Geometry: final body of the model. Coordinates: model frame, mm. Face numbers are marked on the shaded views. A direction names the side the tool comes from. Give positions to 0.01 mm unless a question says otherwise; leave off trailing zeros. Write each loop counter-clockwise with the first axis right and the second up, starting at its lowest first coordinate (ties: lowest second). Pieces come first, ordered by that corner, then holes.
Q1. Section A-A (x = 60.5). Return the cut outline in (y, z), plus the area to 3 significant figures.
Q2. Line query: line 1 (Y direction, x = 60.5, z = 2.9); line 2 (X direction, y = -88.6, z = -52.57); line 3 (Z direction, x = 18.5, y = -48). Output: solid intervals per line, ascending.
Q3. Mould query, pull axis Z, two halves, no side actions, for the marked faces 4, 5 and 6. Classes: +Z half, -Z half, draft (parallel to the pull), parting line (faces both ways), or undercut.
Q4. Pin query (flat end, axial travel): pin 1 Ø4 at (y, z) = (-19, 3.5) entering from -X; pin 2 Ø1.5 at (x, y) = (25, -57) entering from -Z; pin 3 Ø9.5 at (x, z) = (42, -31.5) entering from -Y; pin 4 Ø6.5 at (x, y) = (60.5, -22.94) entering from -Z. Return the tip coordinate at first contact, or that it passes through.
Q5. Reachability of the marked faces 1, 2 and 3 from +Z, -Z, +X, -X, +Y, -Y: full face, straight path, thin tool, end or side. Return the list, or none.
Q6. Section D-D (y = -50.5). Return the cut outline in (x, z).
Q7. Section C-C (y = -35.5). Return the cut outline in (x, z).
Q8. Section B-B (z = -21.66). Return the cut outline in (x, y).
from build123d import *

# Parameters (mm, degrees)
BOSS_EXTRUDE1_DEPTH   = 5
SKETCH2_W             = 6.35
SKETCH2_H             = 50
BOSS_EXTRUDE2_DEPTH   = 52.48
CUT_EXTRUDE1_REACH    = 106.448
SKETCH3_R             = 20.44
SKETCH3_R_2           = 2.555
SKETCH3_W             = 5
SKETCH3_H             = 50
CUT_EXTRUDE2_REACH    = 108.104
SKETCH4_R             = 3.5
CUT_EXTRUDE6_REACH    = 108.104
SKETCH14_W            = 23.196263878
SKETCH14_H            = 15.316152196
SKETCH15_W            = 12
SKETCH15_H            = 3.2
BOSS_EXTRUDE7_DEPTH   = 46.5
BOSS_EXTRUDE8_REACH   = 98.667
SKETCH16_W            = 12
SKETCH16_H            = 3.5
SKETCH17_W            = 12
SKETCH17_H            = 3.5
BOSS_EXTRUDE9_DEPTH   = 15
CHAMFER2_SIZE         = 2
SKETCH22_W            = 12
SKETCH22_H            = 15
BOSS_EXTRUDE10_DEPTH  = 0.72
CUT_EXTRUDE8_REACH    = 103.606
CUT_EXTRUDE7_REACH    = 120.762
SKETCH18_R            = 3.25
MIRROR2_OUTLINE_W     = 50
MIRROR2_OUTLINE_H     = 5
MIRROR2_DEPTH         = 68
MIRROR2_2_OUTLINE_R   = 2.555
MIRROR2_2_OUTLINE_R_2 = 20.44
MIRROR2_2_DEPTH       = 6.35
MIRROR2_START         = 37.56
MIRROR2_3_DEPTH       = 12
MIRROR2_START_2       = 51
MIRROR2_4_OUTLINE_W   = 13.938985111
MIRROR2_4_OUTLINE_H   = 5
MIRROR2_4_DEPTH       = 5.9999999
MIRROR2_START_3       = 64.0000001
MIRROR2_5_OUTLINE_W   = 13.938985111
MIRROR2_5_OUTLINE_H   = 5
MIRROR2_5_DEPTH       = 5.9999999
MIRROR2_6_DEPTH       = 5
BOSS_EXTRUDE11_DEPTH  = 12
CUT_EXTRUDE9_REACH    = 132.799
SKETCH26_W            = 121.241742099
SKETCH26_H            = 103.992632166
SKETCH27_R            = 3.25
CUT_EXTRUDE10_DEPTH   = 119.762181294


with BuildPart() as part:
    # Sketch1 → Boss-Extrude1 (new body)
    with BuildSketch(Plane.XY):
        Polygon((0, 0), (0, 50), (51, 50), (51, 64.061014889), (70, 64.061014889), (70, -13.938985111), (51, -13.938985111), (51, 0), align=None)
    extrude(amount=BOSS_EXTRUDE1_DEPTH)

    # Sketch2 → Boss-Extrude2 (add)
    with BuildSketch(Plane(origin=(0, 0, 0), x_dir=(-1, 0, 0), z_dir=(0, 0, -1))):
        with Locations((-3.175, 25)):
            Rectangle(SKETCH2_W, SKETCH2_H)
    extrude(amount=BOSS_EXTRUDE2_DEPTH)

    # Sketch3 → Cut-Extrude1 (cut, up to next)
    with BuildSketch(Plane(origin=(6.35, 0, 0), x_dir=(0, 0, -1), z_dir=(1, 0, 0)), mode=Mode.PRIVATE) as cut_extrude1_sk1:
        with Locations((21.66, 25)):
            Circle(SKETCH3_R)
    cut_extrude1_tool1 = extrude(cut_extrude1_sk1.sketch, amount=-CUT_EXTRUDE1_REACH, mode=Mode.PRIVATE) & part.part
    # Sketch3 → Cut-Extrude1 (cut, up to next)
    with BuildSketch(Plane(origin=(6.35, 0, 0), x_dir=(0, 0, -1), z_dir=(1, 0, 0)), mode=Mode.PRIVATE) as cut_extrude1_sk2:
        with Locations((3.695, 42.955)):
            Circle(SKETCH3_R_2)
    cut_extrude1_tool2 = extrude(cut_extrude1_sk2.sketch, amount=-CUT_EXTRUDE1_REACH, mode=Mode.PRIVATE) & part.part
    # Sketch3 → Cut-Extrude1 (cut, up to next)
    with BuildSketch(Plane(origin=(6.35, 0, 0), x_dir=(0, 0, -1), z_dir=(1, 0, 0)), mode=Mode.PRIVATE) as cut_extrude1_sk3:
        with Locations((39.615, 7.045)):
            Circle(SKETCH3_R_2)
    cut_extrude1_tool3 = extrude(cut_extrude1_sk3.sketch, amount=-CUT_EXTRUDE1_REACH, mode=Mode.PRIVATE) & part.part
    # Sketch3 → Cut-Extrude1 (cut, up to next)
    with BuildSketch(Plane(origin=(6.35, 0, 0), x_dir=(0, 0, -1), z_dir=(1, 0, 0)), mode=Mode.PRIVATE) as cut_extrude1_sk4:
        with Locations((49.98, 25)):
            Rectangle(SKETCH3_W, SKETCH3_H)
    cut_extrude1_tool4 = extrude(cut_extrude1_sk4.sketch, amount=-CUT_EXTRUDE1_REACH, mode=Mode.PRIVATE) & part.part
    add(cut_extrude1_tool1.solids().sort_by_distance((6.35, 25, -21.66))[0], mode=Mode.SUBTRACT)
    add(cut_extrude1_tool2.solids().sort_by_distance((6.35, 42.955, -3.695))[0], mode=Mode.SUBTRACT)
    add(cut_extrude1_tool3.solids().sort_by_distance((6.35, 7.045, -39.615))[0], mode=Mode.SUBTRACT)
    add(cut_extrude1_tool4.solids().sort_by_distance((6.35, 25, -49.98))[0], mode=Mode.SUBTRACT)

    # Sketch4 → Cut-Extrude2 (cut, up to next)
    with BuildSketch(Plane(origin=(0, 0, 0), x_dir=(-1, 0, 0), z_dir=(0, 0, -1)), mode=Mode.PRIVATE) as cut_extrude2_sk1:
        with Locations((-60.5, 55.061014889)):
            Circle(SKETCH4_R)
    cut_extrude2_tool1 = extrude(cut_extrude2_sk1.sketch, amount=-CUT_EXTRUDE2_REACH, mode=Mode.PRIVATE) & part.part
    # Sketch4 → Cut-Extrude2 (cut, up to next)
    with BuildSketch(Plane(origin=(0, 0, 0), x_dir=(-1, 0, 0), z_dir=(0, 0, -1)), mode=Mode.PRIVATE) as cut_extrude2_sk2:
        with Locations((-60.5, -4.938985111)):
            Circle(SKETCH4_R)
    cut_extrude2_tool2 = extrude(cut_extrude2_sk2.sketch, amount=-CUT_EXTRUDE2_REACH, mode=Mode.PRIVATE) & part.part
    add(cut_extrude2_tool1.solids().sort_by_distance((60.5, 55.061015, 0))[0], mode=Mode.SUBTRACT)
    add(cut_extrude2_tool2.solids().sort_by_distance((60.5, -4.938985, 0))[0], mode=Mode.SUBTRACT)

    # Sketch14 → Cut-Extrude6 (cut, up to next)
    with BuildSketch(Plane(origin=(0, 0, 0), x_dir=(-1, 0, 0), z_dir=(0, 0, -1)), mode=Mode.PRIVATE) as cut_extrude6_sk1:
        with Locations((-62.598131939, 57.658076098)):
            Rectangle(SKETCH14_W, SKETCH14_H)
    cut_extrude6_tool1 = extrude(cut_extrude6_sk1.sketch, amount=-CUT_EXTRUDE6_REACH, mode=Mode.PRIVATE) & part.part
    add(cut_extrude6_tool1.solids().sort_by_distance((62.598132, 57.658076, 0))[0], mode=Mode.SUBTRACT)

    # Sketch15 → Boss-Extrude7 (add)
    with BuildSketch(Plane(origin=(0, 0, 0), x_dir=(-1, 0, 0), z_dir=(0, 0, -1))):
        with Locations((-43.56, 1.6)):
            Rectangle(SKETCH15_W, SKETCH15_H)
    extrude(amount=BOSS_EXTRUDE7_DEPTH)

    # Boss-Extrude8: up to this plane
    boss_extrude8_end = Plane(origin=(166.832994776, 64.085435133, -66.619565524), z_dir=(-1.1416993347548052e-15, 0.9990256874715413, 0.04413247978546202))
    # Sketch16 → Boss-Extrude8 (add, up to the surface)
    with BuildSketch(Plane(origin=(0, 3.2, 0), x_dir=(1, 0, 0), z_dir=(0, 1, 0)), mode=Mode.PRIVATE) as boss_extrude8_sk1:
        with Locations((43.56, 44.75)):
            Rectangle(SKETCH16_W, SKETCH16_H)
    boss_extrude8_tool1 = split(extrude(boss_extrude8_sk1.sketch, amount=BOSS_EXTRUDE8_REACH, mode=Mode.PRIVATE), bisect_by=boss_extrude8_end, keep=Keep.BOTH, mode=Mode.PRIVATE)
    add(boss_extrude8_tool1.solids().sort_by_distance((43.56, 3.2, -44.75))[0])

    # Sketch17 → Boss-Extrude9 (add)
    with BuildSketch(Plane(origin=(0, 0, -46.5), x_dir=(-1, 0, 0), z_dir=(0, 0, -1))):
        with Locations((-43.56, 61.446642853)):
            Rectangle(SKETCH17_W, SKETCH17_H)
    extrude(amount=BOSS_EXTRUDE9_DEPTH)

    # Chamfer2
    chamfer2_edges = [part.edges().sort_by_distance(p)[0] for p in [
        (3.175, 0, -47.48),
        (3.175, 50, -47.48),
        (70, 50, 2.5),
    ]]
    chamfer(chamfer2_edges, length=CHAMFER2_SIZE)

    # Sketch22 → Boss-Extrude10 (add)
    with BuildSketch(Plane(origin=(0, 63.196642853, 0), x_dir=(1, 0, 0), z_dir=(0, 1, 0))):
        with Locations((43.56, 54)):
            Rectangle(SKETCH22_W, SKETCH22_H)
    extrude(amount=BOSS_EXTRUDE10_DEPTH)

    # Sketch23 → Cut-Extrude8 (cut, up to next)
    with BuildSketch(Plane(origin=(49.56, 0, 0), x_dir=(0, 0, -1), z_dir=(1, 0, 0)), mode=Mode.PRIVATE) as cut_extrude8_sk1:
        Polygon((46.5, 63.916642853), (46.5, 63.196642853), (61.5, 63.916642853), align=None)
    cut_extrude8_tool1 = extrude(cut_extrude8_sk1.sketch, amount=-CUT_EXTRUDE8_REACH, mode=Mode.PRIVATE) & part.part
    add(cut_extrude8_tool1.solids().sort_by_distance((49.56, 63.676643, -51.5))[0], mode=Mode.SUBTRACT)

    # Cut-Extrude7: up to this plane
    cut_extrude7_end = Plane(origin=(-0.001, 63.196642853, -46.5), z_dir=(-2.1659106514416256e-15, -0.9988499868416298, -0.04794479936839813))
    # Sketch18 → Cut-Extrude7 (cut, up to the surface)
    with BuildSketch(Plane.XZ.offset(-59.696642853), mode=Mode.PRIVATE) as cut_extrude7_sk1:
        with Locations(Location((43.56, -52.57, 0), (0, 0, 270))):
            Circle(SKETCH18_R)
    cut_extrude7_tool1 = split(extrude(cut_extrude7_sk1.sketch, amount=-CUT_EXTRUDE7_REACH, mode=Mode.PRIVATE), bisect_by=cut_extrude7_end, keep=Keep.BOTH, mode=Mode.PRIVATE)
    add(cut_extrude7_tool1.solids().sort_by_distance((43.56, 59.696643, -52.57))[0], mode=Mode.SUBTRACT)



with BuildPart() as body_2:
    # Mirror2: read off the stored shape, not the designer's step
    # Mirror2 outline → Mirror2 (new body)
    with BuildSketch(Plane.YZ):
        with Locations((-52.877970222, 2.5)):
            Rectangle(MIRROR2_OUTLINE_W, MIRROR2_OUTLINE_H)
    extrude(amount=MIRROR2_DEPTH)

    # Mirror2 2 outline → Mirror2 2 (add)
    with BuildSketch(Plane.YZ):
        Polygon((-27.877970222, -45.48), (-27.877970222, 0), (-77.877970222, 0), (-77.877970222, -45.48), (-75.877970222, -47.48), (-29.877970222, -47.48), align=None)
        with Locations((-34.922970222, -39.615)):
            Circle(MIRROR2_2_OUTLINE_R, mode=Mode.SUBTRACT)
        with Locations((-70.832970222, -3.695)):
            Circle(MIRROR2_2_OUTLINE_R, mode=Mode.SUBTRACT)
        with Locations((-52.877970222, -21.66)):
            Circle(MIRROR2_2_OUTLINE_R_2, mode=Mode.SUBTRACT)
    extrude(amount=MIRROR2_2_DEPTH)


with BuildPart() as part_1:
    add(part.part)

    add(body_2.part)  # Mirror2 3 merges body 2
    # Mirror2 3 outline → Mirror2 3 (add)
    with BuildSketch(Plane.YZ.offset(MIRROR2_START)):
        Polygon((-31.077970222, -46.5), (0, -46.5), (0, -43), (-27.877970222, -43), (-27.877970222, 0), (-31.077970222, 0), align=None)
    extrude(amount=MIRROR2_3_DEPTH)

    # Mirror2 4 outline → Mirror2 4 (add)
    with BuildSketch(Plane.YZ.offset(MIRROR2_START_2)):
        with Locations((-20.908477667, 2.5)):
            Rectangle(MIRROR2_4_OUTLINE_W, MIRROR2_4_OUTLINE_H)
    extrude(amount=MIRROR2_4_DEPTH)

    # Mirror2 5 outline → Mirror2 5 (add)
    with BuildSketch(Plane.YZ.offset(MIRROR2_START_3)):
        with Locations((-20.908477667, 2.5)):
            Rectangle(MIRROR2_5_OUTLINE_W, MIRROR2_5_OUTLINE_H)
    extrude(amount=MIRROR2_5_DEPTH)

    # Mirror2 6 outline → Mirror2 6 (add)
    with BuildSketch(Plane.XY):
        Polygon((70, -75.877970222), (70, -27.877970222), (68, -27.877970222), (68, -77.877970222), align=None)
        with BuildLine():
            Line((64.0000001, -27.877970222), (64, -22.938985111))
            ThreePointArc((64, -22.938985111), (60.5, -26.438985111), (57, -22.938985111))
            Line((57, -22.938985111), (56.9999999, -27.877970222))
            Line((56.9999999, -27.877970222), (64.0000001, -27.877970222))
        make_face()
        with BuildLine():
            ThreePointArc((57, -22.938985111), (60.5, -19.438985111), (64, -22.938985111))
            Line((64, -22.938985111), (64.0000001, -13.938985111))
            Line((64.0000001, -13.938985111), (56.9999999, -13.938985111))
            Line((56.9999999, -13.938985111), (57, -22.938985111))
        make_face()
    extrude(amount=MIRROR2_6_DEPTH)

    # Sketch25 → Boss-Extrude11 (add)
    with BuildSketch(Plane(origin=(49.56, 0, 0), x_dir=(0, 0, -1), z_dir=(1, 0, 0))):
        Polygon((43, -13.938985111), (46.5, -13.938985111), (46.5, -87.574613075), (61.5, -87.574613075), (61.5, -91.794613075), (46.5, -91.074613075), (43, -90.919998753), (43, -31.077970222), align=None)
    extrude(amount=-BOSS_EXTRUDE11_DEPTH)

    # Cut-Extrude9: up to this face of the body (flat: up to its plane)
    cut_extrude9_end = Plane(part_1.part.faces().sort_by_distance((0, 0.724855186, -20.24))[0])
    # Sketch26 → Cut-Extrude9 (cut, up to the picked face)
    with BuildSketch(Plane(origin=(70, 0, 0), x_dir=(0, 0, -1), z_dir=(1, 0, 0)), mode=Mode.PRIVATE) as cut_extrude9_sk1:
        with Locations((55.62087105, 38.057330972)):
            Rectangle(SKETCH26_W, SKETCH26_H)
    cut_extrude9_tool1 = split(extrude(cut_extrude9_sk1.sketch, amount=-CUT_EXTRUDE9_REACH, mode=Mode.PRIVATE), bisect_by=cut_extrude9_end, keep=Keep.BOTH, mode=Mode.PRIVATE)
    add(cut_extrude9_tool1.solids().sort_by(Axis((70, 38.057331, -55.620871), (-1, 0, 0)))[0], mode=Mode.SUBTRACT)

    # Sketch27 → Cut-Extrude10 (cut, through all)
    with BuildSketch(Plane(origin=(0, -87.574613075, 0), x_dir=(1, 0, 0), z_dir=(0, 1, 0))):
        with Locations(Location((43.56, 52.57, 0), (0, 0, 180))):
            Circle(SKETCH27_R)
    extrude(amount=-CUT_EXTRUDE10_DEPTH, mode=Mode.SUBTRACT)


solid = part_1.part
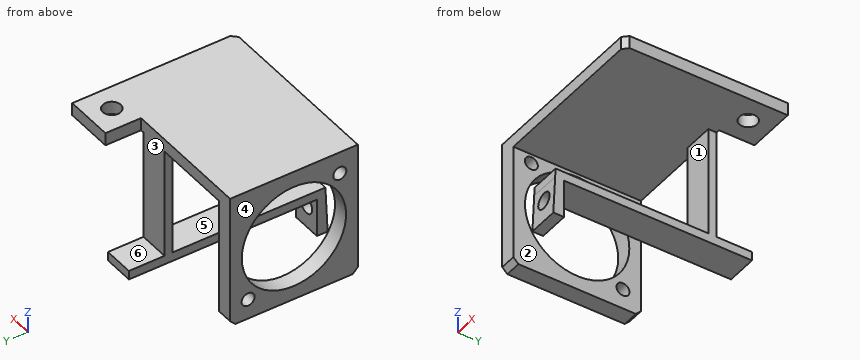
Computed:
1. outline: (-77.88, 0) - (-26.44, 0) - (-26.44, 5) - (-77.88, 5) - close; (-19.44, 0) - (-13.94, 0) - (-13.94, 5) - (-19.44, 5) - close
1. area: 285 mm2
2. line 1: y = -77.88 to -26.44, -19.44 to -13.94
2. line 2: x = 37.56 to 40.31, 46.81 to 49.56
2. line 3: z = 0 to 5
3. face 4: draft
3. face 5: undercut
3. face 6: +Z half
4. pin 1: stops at x = 51
4. pin 2: stops at z = 0
4. pin 3: stops at y = -31.08
4. pin 4: passes through
5. face 1: +X, -Y
5. face 2: -Z, +Y, -Y
5. face 3: +Z, -X, +Y
6. outline: (0, -47.48) - (6.35, -47.48) - (6.35, -41.96) - (0, -41.96) - close; (0, -1.36) - (6.35, -1.36) - (6.35, 0) - (70, 0) - (70, 5) - (0, 5) - close; (37.56, -46.5) - (49.56, -46.5) - (49.56, -43) - (37.56, -43) - close
7. outline: (0, -47.48) - (6.35, -47.48) - (6.35, -42.1) - (0, -42.1) - close; (0, -37.13) - (6.35, -37.13) - (6.35, -32.42) - (0, -32.42) - close; (0, -10.9) - (6.35, -10.9) - (6.35, 0) - (70, 0) - (70, 5) - (0, 5) - close; (37.56, -46.5) - (49.56, -46.5) - (49.56, -43) - (37.56, -43) - close
8. outline: (0, -77.88) - (6.35, -77.88) - (6.35, -73.32) - (0, -73.32) - close; (0, -32.44) - (6.35, -32.44) - (6.35, -27.88) - (0, -27.88) - close; (37.56, -31.08) - (49.56, -31.08) - (49.56, -27.88) - (37.56, -27.88) - close
